Verification items for this drawing (mm, ordinates from the low corner). Round coordinates to 2 decimals unless told otherwise and drop trailing zeros. Order: outer loops, then holes, each group sorted by start corner. A loop starts at its lowest first (then second) coordinate and runs counter-clockwise, first axis right, second up. Notation, with made-up numbers: (85.5, -24) - (133.5, -24) arc R7 cw to (133.5, -20) - close; hole circle Ø2 at (4, 3). An arc over 180 degrees is marked (long way). Answer as CSV lines item,"result". Start each with the question number.
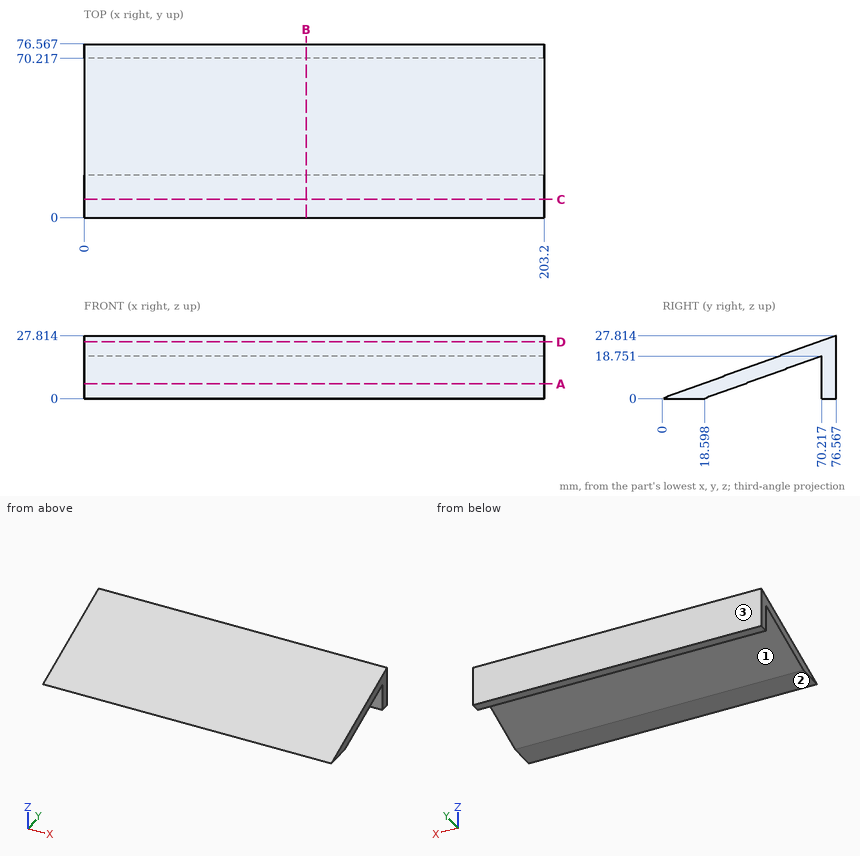
1. Thickness scan on probe 1 along Z at (x, y) = (134, 9); probe 2 along Z at (x, y) = (36.5, 57.5). Record the ranges inside material, lowest first.
2. Section check C-C on y = 8. Record the boundary of the cut face in (x, z).
3. Go/stop test with flat-tipped pins: pin 1 Ø4 at (x, y) = (180.5, 67.5) entering from -Z; pin 2 Ø4 at (x, y) = (116, 11) entering from +Z; pin 3 Ø3 at (x, y) = (138, 47.5) entering from -Z (1 decimal). Record where each tip stops, or that it passes through.
4. Section check D-D on z = 25. Record the boundary of the cut face in (x, y).
5. Draft check along Y on the marked faces 1, 2 and 3. Enter one of: released by +Y, released by -Y, zero draft, split by the parting line, or undercut.
6. Section check A-A on z = 6.5. Record the boundary of the cut face in (x, y), plus the area to 3 significant figures.
7. Section check B-B on x = 98. Record the boundary of the cut face in (y, z), plus the area to 3 significant figures.
Numbers:
1,probe 1,"z = 0 to 3.27"
1,probe 2,"z = 14.13 to 20.89"
2,outline,"(0, 0) - (203.2, 0) - (203.2, 2.91) - (0, 2.91) - close"
3,pin 1,"stops at z = 17.04"
3,pin 2,"stops at z = 4.72"
3,pin 3,"stops at z = 10"
4,outline,"(0, 68.82) - (203.2, 68.82) - (203.2, 76.57) - (0, 76.57) - close"
5,face 1,"undercut"
5,face 2,"zero draft"
5,face 3,"released by +Y"
6,outline,"(0, 17.89) - (203.2, 17.89) - (203.2, 36.49) - (0, 36.49) - close; (0, 70.22) - (203.2, 70.22) - (203.2, 76.57) - (0, 76.57) - close"
6,area,"5,070 mm2"
7,outline,"(0, 0) - (18.6, 0) - (70.22, 18.75) - (70.22, 0) - (76.57, 0) - (76.57, 27.81) - close"
7,area,"581 mm2"
